```python
from build123d import *

# Parameters (mm, degrees)
SKETCH1_W            = 70.2
SKETCH1_H            = 50.2
SKETCH1_W_2          = 66.2
SKETCH1_H_2          = 46.2
BOSS_EXTRUDE1_DEPTH  = 1.25
SKETCH2_W            = 70.2
SKETCH2_H            = 50.2
SKETCH2_W_2          = 36
SKETCH2_H_2          = 30
BOSS_EXTRUDE2_DEPTH  = 1
SKETCH15_W           = 70.2
SKETCH15_H           = 50.2
SKETCH15_W_2         = 66.2
SKETCH15_H_2         = 46.2
BOSS_EXTRUDE3_DEPTH  = 1.75
CUT_SWEEP2_PROFILE_R = 0.5
FILLET2_R            = 0.1


with BuildPart() as part:
    # Sketch1 → Boss-Extrude1 (new body)
    with BuildSketch(Plane(origin=(0, 0, 0), x_dir=(1, 0, 0), z_dir=(0, 1, 0))):
        Rectangle(SKETCH1_W, SKETCH1_H)
        Rectangle(SKETCH1_W_2, SKETCH1_H_2, mode=Mode.SUBTRACT)
    extrude(amount=BOSS_EXTRUDE1_DEPTH)

    # Sketch2 → Boss-Extrude2 (add)
    with BuildSketch(Plane(origin=(0, 1.25, 0), x_dir=(1, 0, 0), z_dir=(0, 1, 0))):
        Rectangle(SKETCH2_W, SKETCH2_H)
        Rectangle(SKETCH2_W_2, SKETCH2_H_2, mode=Mode.SUBTRACT)
    extrude(amount=BOSS_EXTRUDE2_DEPTH)

    # Sketch15 → Boss-Extrude3 (add)
    with BuildSketch(Plane.XZ):
        Rectangle(SKETCH15_W, SKETCH15_H)
        Rectangle(SKETCH15_W_2, SKETCH15_H_2, mode=Mode.SUBTRACT)
    extrude(amount=BOSS_EXTRUDE3_DEPTH)

    # Cut-Sweep2: sweep along a path in Sketch3
    with BuildLine(Plane(origin=(0, -0.85, 0), x_dir=(-1, 0, 0), z_dir=(0, -1, 0))) as cut_sweep2_path:
        Line((-33.1, 23.1), (33.1, 23.1))
        Line((33.1, 23.1), (33.1, -23.1))
        Line((33.1, -23.1), (-33.1, -23.1))
        Line((-33.1, -23.1), (-33.1, 23.1))
    # Cut-Sweep2 profile (on start of the path) → Cut-Sweep2 (sweep, cut)
    with BuildSketch(Plane(origin=(33.1, -0.85, -23.1), x_dir=(0, 0, -1), z_dir=(-1, 0, 0))):
        Circle(CUT_SWEEP2_PROFILE_R)
    sweep(path=cut_sweep2_path.line, transition=Transition.RIGHT, mode=Mode.SUBTRACT)

    # Fillet2
    fillet2_edges = [part.edges().sort_by_distance(p)[0] for p in [
        (0, -0.35, -23.1),
        (0, -1.35, -23.1),
        (0, -1.35, 23.1),
        (0, -0.35, 23.1),
        (-33.1, -1.35, 0),
        (-33.1, -0.35, 0),
        (33.1, -1.35, 0),
        (33.1, -0.35, 0),
    ]]
    fillet(fillet2_edges, radius=FILLET2_R)


solid = part.part
```
Here's how the part is built. I have some questions about the finished solid (model axes, mm). A direction names the side the tool comes from. Give positions to 0.01 mm unless a question says otherwise; leave off trailing zeros. Write each loop counter-clockwise with the first axis right and the second up, starting at its lowest first coordinate (ties: lowest second). Pieces come first, ordered by that corner, then holes. Notation, with made-up numbers: (11.25, 43) -> (15.25, 43) arc R17 cw to (15.25, 53) -> close; hole circle Ø1 at (83.5, 52.25). An arc over 180 degrees is marked (long way). Use one line per item in the form item = value.
1) We'd pull the mould along X, two halves only. Please class faces 1 (the face through (0, 1, 23.1)), 2 (the face through (-3, -1.75, -24)), 3 (the face through (35.1, 0, 0)): +X half, -X half, draft (parallel to the pull), parting line (faces both ways), or undercut.
Verdict:
face_1 = undercut
face_2 = draft
face_3 = +X half
2) Suppose I cut it at D-D (x = -28.5). Please give me the cut outline in (y, z), and give its area (3 significant figures).
Verdict:
outline = (-1.75, -25.1) -> (2.25, -25.1) -> (2.25, 25.1) -> (-1.75, 25.1) -> (-1.75, 23.1) -> (-1.44, 23.1) arc R0.1 ccw to (-1.34, 23.18) arc R0.5 cw to (-0.36, 23.18) arc R0.1 ccw to (-0.26, 23.1) -> (1.25, 23.1) -> (1.25, -23.1) -> (-0.26, -23.1) arc R0.1 ccw to (-0.36, -23.18) arc R0.5 cw to (-1.34, -23.18) arc R0.1 ccw to (-1.44, -23.1) -> (-1.75, -23.1) -> close
area = 61.4 mm2
3) On a 3-axis mill with a long thin cutter (end or side, diameter ignored), from which of +Z, -Z, +X, -X, +Y, -Y can I reach the whole of each face in a straight line? I mean faces 4 (the face through (0, 1.25, -16)), 5 (the face through (0, 0, 25.1)). Say none if no direction works.
Verdict:
face_4 = -Y
face_5 = +Z, +X, -X, +Y, -Y
4) Suppose I cut it at B-B (x = 8). Please give me the cut outline in (y, z), and give its area (3 significant figures).
Verdict:
outline = (-1.75, -25.1) -> (2.25, -25.1) -> (2.25, -15) -> (1.25, -15) -> (1.25, -23.1) -> (-0.26, -23.1) arc R0.1 ccw to (-0.36, -23.18) arc R0.5 cw to (-1.34, -23.18) arc R0.1 ccw to (-1.44, -23.1) -> (-1.75, -23.1) -> close; (-1.75, 23.1) -> (-1.44, 23.1) arc R0.1 ccw to (-1.34, 23.18) arc R0.5 cw to (-0.36, 23.18) arc R0.1 ccw to (-0.26, 23.1) -> (1.25, 23.1) -> (1.25, 15) -> (2.25, 15) -> (2.25, 25.1) -> (-1.75, 25.1) -> close
area = 31.4 mm2
5) If I drill on L1, parallel to Z at x = 1, y = -0.2; L2, parallel to X at y = -0.9, z = -7.5; L3, parallel to X at y = 0.75, z = 20, over which ranges is the centre line in solid material (lowest first)? Write a range as [from, to].
Verdict:
L1 = [-25.1, -23.1], [23.1, 25.1]
L2 = [-35.1, -33.6], [33.6, 35.1]
L3 = [-35.1, -33.1], [33.1, 35.1]
6) Suppose I cut it at C-C (y = 0.55). Please give me the cut outline in (x, z).
Verdict:
outline = (-35.1, -25.1) -> (35.1, -25.1) -> (35.1, 25.1) -> (-35.1, 25.1) -> close; hole (-33.1, -23.1) -> (33.1, -23.1) -> (33.1, 23.1) -> (-33.1, 23.1) -> close
7) Suppose I cut it at A-A (z = 6.5). Please give me the cut outline in (x, y).
Verdict:
outline = (-35.1, -1.75) -> (-33.1, -1.75) -> (-33.1, -1.44) arc R0.1 ccw to (-33.18, -1.34) arc R0.5 cw to (-33.18, -0.36) arc R0.1 ccw to (-33.1, -0.26) -> (-33.1, 1.25) -> (-18, 1.25) -> (-18, 2.25) -> (-35.1, 2.25) -> close; (18, 1.25) -> (33.1, 1.25) -> (33.1, -0.26) arc R0.1 ccw to (33.18, -0.36) arc R0.5 cw to (33.18, -1.34) arc R0.1 ccw to (33.1, -1.44) -> (33.1, -1.75) -> (35.1, -1.75) -> (35.1, 2.25) -> (18, 2.25) -> close
8) I'm going to push flat-ended pins straight in: pin 1 (3 mm diameter, centred on x = -16, z = 9, fed in from -Y); pin 2 (23 mm diameter, centred on x = -0.5, z = -5, fed in from -Y). Where does each tip first touch, or does it pass through?
Verdict:
pin_1 = through
pin_2 = 1.25
